The drawing under review shows one solid part. Ordinate dimensions are in mm from its lowest x, y, z. Coordinates: 2 decimals unless noted, no trailing zeros. Write each loop counter-clockwise with the first axis right and the second up, starting at its lowest first coordinate (ties: lowest second). Pieces come first, ordered by that corner, then holes.
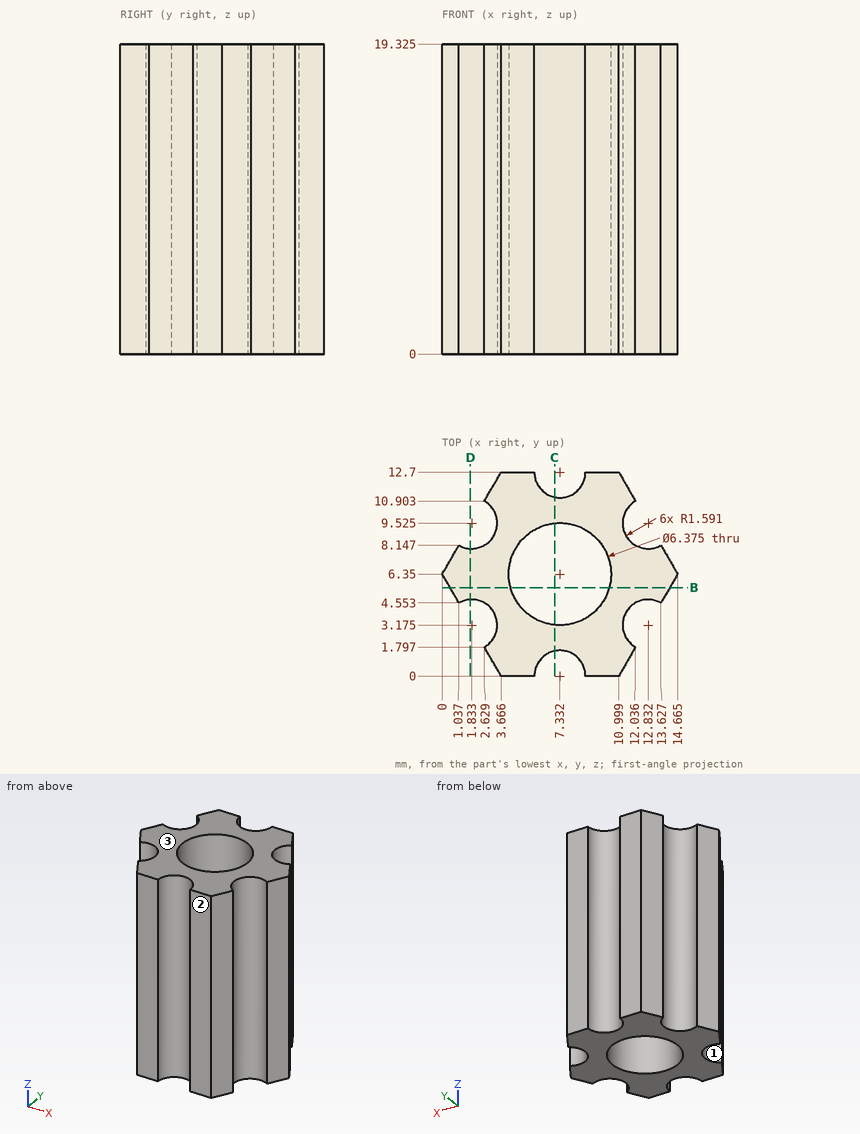
1) For L1, parallel to Y at x = 11.75, z = 17 (1 decimal); L2, parallel to Y at x = 5, z = 15.75 (1 decimal); L3, parallel to Y at x = 8.25, z = 6.5 (1 decimal), list the stretches that pass through material, from the lowest coordinate up.
2) Consider section C-C (x = 7). Give the boundary of the cut face in (y, z) (1 decimal).
3) Consider section D-D (x = 1.75). Give the boundary of the cut face in (y, z) (1 decimal).
4) The part is to be moulded in two halves that separate along Y. For the marked faces 1, 2 and 3, say which applies: pulls with the +Y half, pulls with the -Y half, needs draft (parallel to the pull), parting line crosses it, or undercut.
5) Clearance check with flat-ended pins moving along their axes: P1, Ø6, axis at y = 10.5, z = 14, coming from the +X side; P2, Ø2, axis at y = 4, z = 10.5, coming from the +X side (1 decimal); P3, Ø6, axis at x = 1.5, z = 7, coming from the -Y side; P4, Ø1.5, axis at y = 3.5, z = 3.5, coming from the +X side. State where each tip first meets the part, or that it passes through.
6) Consider section B-B (y = 5.5). Give the boundary of the cut face in (x, z) (1 decimal).
Results:
1. L1: y = 1.3 to 2, 4.3 to 8.4, 10.7 to 11.4
1. L2: y = 0 to 4.2, 8.5 to 12.7
1. L3: y = 1.3 to 3.3, 9.4 to 11.4
2. outline: (1.6, 0) - (3.2, 0) - (3.2, 19.3) - (1.6, 19.3) - close; (9.5, 0) - (11.1, 0) - (11.1, 19.3) - (9.5, 19.3) - close
3. outline: (4.8, 0) - (7.9, 0) - (7.9, 19.3) - (4.8, 19.3) - close
4. face 1: undercut
4. face 2: pulls with the -Y half
4. face 3: needs draft
5. P1: stops at x = 14
5. P2: stops at x = 13.9
5. P3: stops at y = 0
5. P4: stops at x = 11.66
6. outline: (0.5, 0) - (4.3, 0) - (4.3, 19.3) - (0.5, 19.3) - close; (10.4, 0) - (14.2, 0) - (14.2, 19.3) - (10.4, 19.3) - close
